Geometry: see drawing. Coordinates: mm, zero at the bounding-box minimum. A direction names the side the tool comes from. Give positions to 0.01 mm unless a question says otherwise; leave off trailing zeros. Loops run counter-clockwise (first coordinate to the right, second up) from the corner with the lowest first, then second, coordinate; pieces in that order, holes last. Notation, with made-up numbers: M 84.25,13.5 L 104.25,13.5 A17 cw 104.25,23.5 Z; hole C 72.5,24 d3. An arc over 180 degrees is marked long. Put each result on its own line as item: value.
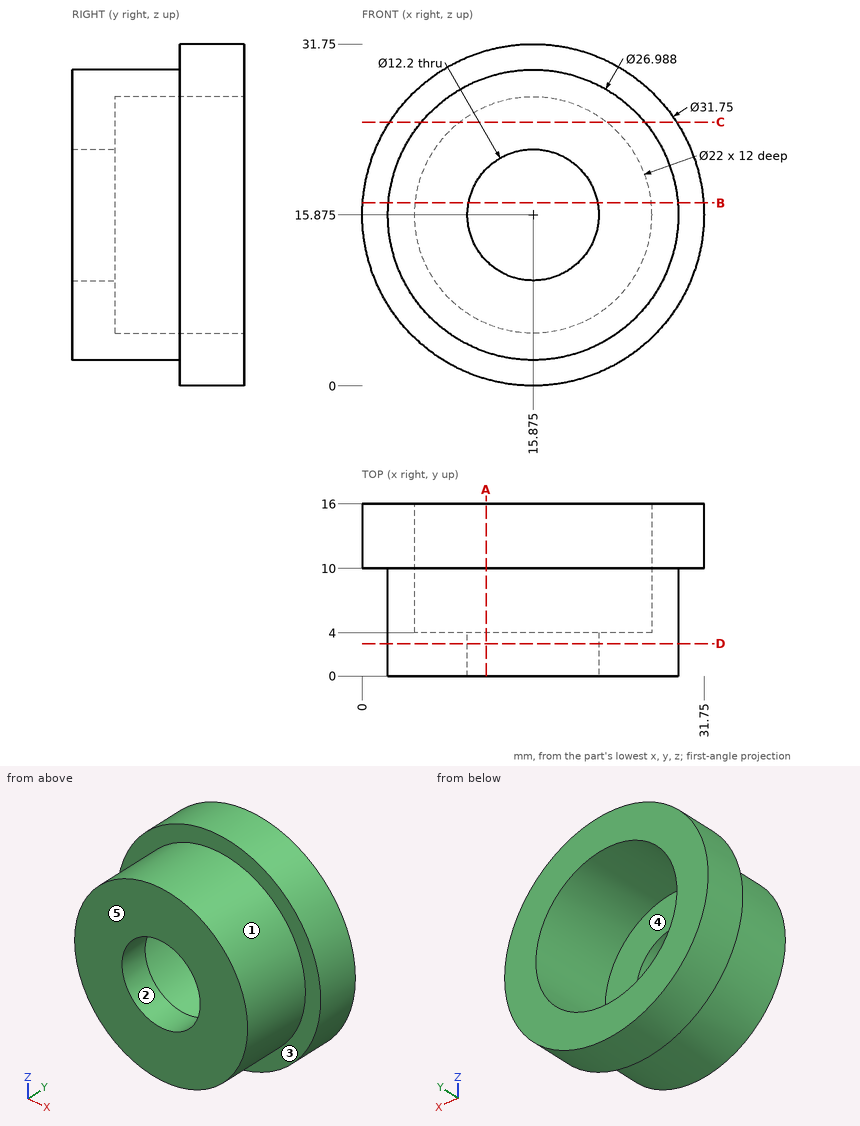
1. Section query C-C (z = 24.5). Output: boundary loops of the cut face in (x, y).
Found:
outline: M 2.55,10 L 5.5,10 L 5.5,0 L 26.25,0 L 26.25,10 L 29.2,10 L 29.2,16 L 22.7,16 L 22.7,4 L 9.05,4 L 9.05,16 L 2.55,16 Z
2. Access query for the marked faces 4 and 5. Directions: +Z, -Z, +X, -X, +Y, -Y. A direction counts if a zero-diameter tool reaches every point of the face in a straight line with its end or side. Return the directions, or none.
Found:
face 4: +Y
face 5: +Z, -Z, +X, -X, -Y
3. Section query B-B (z = 17). Output: boundary loops of the cut face in (x, y).
Found:
outline: M 0.04,10 L 2.43,10 L 2.43,0 L 9.88,0 L 9.88,4 L 4.93,4 L 4.93,16 L 0.04,16 Z; M 21.87,0 L 29.32,0 L 29.32,10 L 31.71,10 L 31.71,16 L 26.82,16 L 26.82,4 L 21.87,4 Z
4. Draft query along X for the marked faces 1, 2 and 3. Return one class per face: pulls with the +X half, pulls with the -X half, needs draft (parallel to the pull), parting line crosses it, or undercut.
Found:
face 1: parting line crosses it
face 2: undercut
face 3: needs draft
5. Contact query for flat-ended pins moving along their axis: P1, Ø13, axis at x = 15.875, z = 15.875, coming from the +Y side; P2, Ø8, axis at x = 22, y = 4, coming from the +Z side; P3, Ø3, axis at y = 2.5, z = 18, coming from the +X side. Output: stop coordinate, or through.
Found:
P1: y = 4
P2: z = 29.2
P3: x = 29.35
6. Section query A-A (x = 11.5). Output: boundary loops of the cut face in (y, z) (1 decimal), plus the area to 3 significant figures.
Found:
outline: M 0,3.1 L 10,3.1 L 10,0.6 L 16,0.6 L 16,5.8 L 4,5.8 L 4,11.6 L 0,11.6 Z; M 0,20.1 L 4,20.1 L 4,26 L 16,26 L 16,31.1 L 10,31.1 L 10,28.6 L 0,28.6 Z
area: 162 mm^2
7. Material intervals for line 1 (X direction, y = 5.5, z = 16) (1 decimal); line 2 (X direction, y = 13.5, z = 21); line 3 (Y direction, x = 3.5, z = 8), sorted ascending. Write a range as from..to.
Found:
line 1: 2.4..4.9, 26.9..29.4
line 2: 0.85..6.14, 25.61..30.9
line 3: 10..16
8. Section query D-D (y = 3). Output: boundary loops of the cut face in (x, z) (1 decimal), plus the area to 3 significant figures.
Found:
outline: C 15.9,15.9 d27; hole C 15.9,15.9 d12.2
area: 455 mm^2
